from build123d import *

# Parameters (mm, degrees)
F0_W           = 51
F0_H           = 47.5
F1_DEPTH       = 4
F2_W           = 43
F2_H           = 43
F2_R           = 11
F3_DEPTH       = 2
F4_DEPTH       = 4.001
F5_D           = 3
F6_R           = 2
F7_W           = 9.5
F7_H           = 32
F8_DEPTH       = 2
F9_D           = 3
F9_CSINK_D     = 6
F9_CSINK_ANGLE = 90
F10_D          = 2.5
F11_R          = 2
F13_R          = 4


# Not quite as in the source:
# - two fillets or chamfers of one size are made in one step
# - a pattern or mirror of a feature is missing from the dataset's text; its kind, count and spacing are read off the source's solid


with BuildPart() as f1:
    # F0 (on Front) → F1 (new body)
    with BuildSketch(Plane.XZ):
        Polygon((25.5, -2), (-25.5, -2), (-30, -2), (-30, -42), (30, -42), (30, -2), align=None)
        with Locations((0, 21.75)):
            Rectangle(F0_W, F0_H)
    extrude(amount=F1_DEPTH)

    # F2 (on face) → F3 (cut)
    with BuildSketch(Plane(origin=(0, 0, 0), x_dir=(-1, 0, 0), z_dir=(0, 1, 0))):
        with Locations((0, 20)):
            Rectangle(F2_W, F2_H)
        with Locations((0, 20)):
            Circle(F2_R, mode=Mode.SUBTRACT)
    extrude(amount=-F3_DEPTH, mode=Mode.SUBTRACT)

    # F2 (on face) → F4 (cut, through all)
    with BuildSketch(Plane(origin=(0, 0, 0), x_dir=(-1, 0, 0), z_dir=(0, 1, 0))):
        with Locations((0, 20)):
            Circle(F2_R)
    extrude(amount=-F4_DEPTH, mode=Mode.SUBTRACT)

    # F5 (through all)
    with Locations(Plane(origin=(0, 0, 0), x_dir=(-1, 0, 0), z_dir=(0, 1, 0))):
        with Locations((-15.5, 35.5), (15.5, 35.5), (15.5, 4.5), (-15.5, 4.5)):
            Hole(F5_D / 2)

    # F6
    f6_edges = [f1.edges().sort_by_distance(p)[0] for p in [
        (21.5, -1, 41.5),
        (-21.5, -1, 41.5),
        (-21.5, -1, -1.5),
        (21.5, -1, -1.5),
    ]]
    fillet(f6_edges, radius=F6_R)

    # F7 (on face) → F8 (cut)
    with BuildSketch(Plane.XZ.offset(4)):
        with BuildLine():
            Line((-16.5, -38), (-16.5, -6))
            Line((-16.5, -6), (-26, -6))
            Line((-26, -6), (-26, -31.75))
            Line((-26, -31.75), (-23.3, -31.75))
            ThreePointArc((-23.3, -31.75), (-21.7090097423, -32.4090097423), (-21.05, -34))
            Line((-21.05, -34), (-21.05, -38))
            Line((-21.05, -38), (-16.5, -38))
        make_face()
        with BuildLine():
            Line((8.5, -38), (8.5, -6))
            Line((8.5, -6), (-8.5, -6))
            Line((-8.5, -6), (-8.5, -31.75))
            Line((-8.5, -31.75), (-4.89, -31.75))
            ThreePointArc((-4.89, -31.75), (-3.2990097423, -32.4090097423), (-2.64, -34))
            Line((-2.64, -34), (-2.64, -38))
            Line((-2.64, -38), (8.5, -38))
        make_face()
        with Locations((21.25, -22)):
            Rectangle(F7_W, F7_H)
    extrude(amount=-F8_DEPTH, mode=Mode.SUBTRACT)

    # F9 (through all)
    with Locations(Plane.XZ.offset(4)):
        with Locations((-12.5, -9.5), (-12.5, -9.5), (-12.5, -34.5), (12.5, -34.5)):
            f9 = CounterSinkHole(F9_D / 2, F9_CSINK_D / 2, counter_sink_angle=F9_CSINK_ANGLE)

    # F9_copies: F9 across plane
    add(f9.mirror(Plane(origin=(0, 0, 0), x_dir=(0, 0, 1), z_dir=(1, 0, 0))), mode=Mode.SUBTRACT)

    # F10 (through all)
    with Locations(Plane.XZ.offset(4)):
        with Locations((-23.3, -34), (-4.89, -34)):
            Hole(F10_D / 2)

    # F11
    f11_edges = [f1.edges().sort_by_distance(p)[0] for p in [
        (-26, -3, -6),
        (26, -3, -6),
        (26, -3, -38),
        (-16.5, -3, -38),
        (8.5, -3, -38),
        (-16.5, -3, -6),
        (8.5, -3, -6),
        (-8.5, -3, -6),
        (16.5, -3, -6),
        (-8.5, -3, -31.75),
        (-25.5, -2, -2),
        (-30, -2, -2),
        (25.5, -2, -2),
        (30, -2, -2),
        (-21.05, -3, -38),
        (-26, -3, -31.75),
        (-2.64, -3, -38),
    ]]
    fillet(f11_edges, radius=F11_R)

    # F13
    f13_edges = [f1.edges().sort_by_distance(p)[0] for p in [
        (25.5, -2, 45.5),
        (-25.5, -2, 45.5),
        (-30, -2, -42),
        (30, -2, -42),
    ]]
    fillet(f13_edges, radius=F13_R)


solid = f1.part
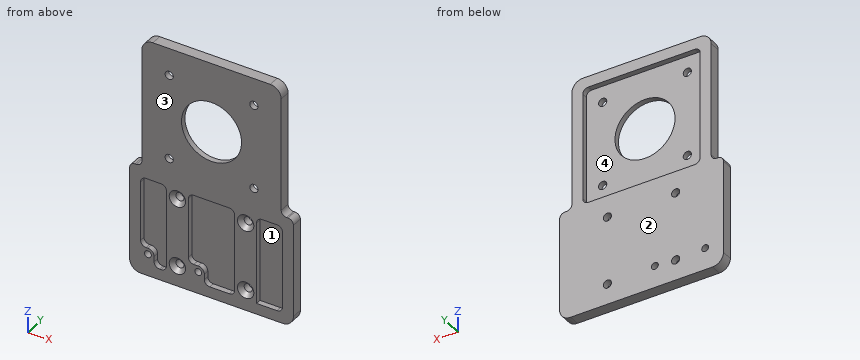
Geometry check sheet. Reference: the model listing, model coordinates, mm. Face numbers are marked on the shaded views. A direction names the side the tool comes from. Give positions to 0.01 mm unless a question says otherwise; leave off trailing zeros. Loops run counter-clockwise (first coordinate to the right, second up) from the corner with the lowest first, then second, coordinate; pieces in that order, holes last. Notation, with made-up numbers: M -9,82 L 23,82 A19 cw 23,110 Z; hole C 34.25,56 d2. An arc over 180 degrees is marked long. Write each question's results on one line, items separated by ' | '.
1) Section check A-A, the plane z = 35.5. Record the boundary of the cut face in (x, y), plus the area to 3 significant figures.
Answers follow:
outline: M -25.5,-4 L -17,-4 L -17,-2 L -21.5,-2 L -21.5,0 L -25.5,0 Z; M -14,-4 L 14,-4 L 14,-2 L -14,-2 Z; M 17,-4 L 25.5,-4 L 25.5,0 L 21.5,0 L 21.5,-2 L 17,-2 Z | area: 106 mm2
2) Thickness scan on line 1 (X direction, y = -1, z = -9.5); line 2 (X direction, y = -3.55, z = -18); line 3 (X direction, y = -1.1, z = 38.5). Record the ranges inside material, lowest first.
Answers follow:
line 1: -30 to -14, -11 to 11, 14 to 30 | line 2: -30 to -26, -16.5 to -8.5, 8.5 to 16.5, 26 to 30 | line 3: -25.5 to -21.5, 21.5 to 25.5
3) Release check for a two-part mould opening along Z. For the marked faces 3 and 4 record: +Z half, -Z half, draft (parallel to the pull), parting line (faces both ways), or undercut.
Answers follow:
face 3: draft | face 4: undercut
4) Section check C-C, the plane y = -1.2. Count the separate pieces of the cut face and the enclosed holes in it, plus the area to 3 significant figures.
Answers follow:
separate pieces: 1 | enclosed holes: 7 | area: 2,930 mm2
5) Section check B-B, the plane x = -12.5. Record the boundary of the cut face in (y, z).
Answers follow:
outline: M -4,-42 L 0,-42 L 0,-36 L -2.5,-36 L -4,-37.5 Z; M -4,-31.5 L -2.5,-33 L 0,-33 L 0,-11 L -2.5,-11 L -4,-12.5 Z; M -4,-6.5 L -2.5,-8 L 0,-8 L 0,-1.5 L -2,-1.5 L -2,41.5 L 0,41.5 L 0,45.5 L -4,45.5 Z
6) Tool access check on the marked faces 1 and 2. Record the directions out of +Z, -Z, +X, -X, +Y, -Y that give a thin tool (end or side, any length) a straight path to the whole face; none if there is none.
Answers follow:
face 1: -Y | face 2: +Z, -Z, +X, -X, +Y
7) Gauge pin test, flat ends, axial feed: pin 1 (2.5 mm diameter, centred on x = -12.5, z = -34.5, fed in from +Y); pin 2 (1 mm diameter, centred on y = -1, z = 29, fed in from +X); pin 3 (1.6 mm diameter, centred on y = -1.5, z = 15, fed in from -X); pin 4 (12 mm diameter, centred on x = -15, z = 33, fed in from +Y). Record the tip position at first contact, or that the pin passes through.
Answers follow:
pin 1: through | pin 2: x = 25.5 | pin 3: x = -25.5 | pin 4: y = -2
